```python
from build123d import *

# Parameters (mm, degrees)
SKETCH_W      = 60
SKETCH_H      = 3
PAD_DEPTH     = 35
SKETCH001_R   = 1.5
SKETCH001_R_2 = 2
SKETCH001_R_3 = 2.25
SKETCH001_R_4 = 1
SKETCH001_W   = 4
SKETCH001_H   = 7
POCKET_DEPTH  = 3


with BuildPart() as part:
    # Sketch → Pad (new body)
    with BuildSketch(Plane.XY):
        with Locations((30, 1.5)):
            Rectangle(SKETCH_W, SKETCH_H)
    extrude(amount=PAD_DEPTH)

    # Sketch001 → Pocket (cut)
    with BuildSketch(Plane.XZ):
        with Locations((22, 10)):
            Circle(SKETCH001_R)
        with Locations((28, 10)):
            Circle(SKETCH001_R_2)
        with Locations((22, 16)):
            Circle(SKETCH001_R_2)
        with Locations((16, 10)):
            Circle(SKETCH001_R_2)
        with Locations((22, 4)):
            Circle(SKETCH001_R_2)
        with Locations((5, 30)):
            Circle(SKETCH001_R_3)
        with Locations((55, 30)):
            Circle(SKETCH001_R_3)
        with Locations((14, 30)):
            Circle(SKETCH001_R_4)
        with Locations((18, 30)):
            Circle(SKETCH001_R_4)
        with Locations((26, 30)):
            Circle(SKETCH001_R_4)
        with Locations((30, 30)):
            Circle(SKETCH001_R_4)
        with Locations((34, 30)):
            Circle(SKETCH001_R_4)
        with Locations((42, 30)):
            Circle(SKETCH001_R_4)
        with Locations((46, 30)):
            Circle(SKETCH001_R_4)
        with Locations((45.6, 15)):
            Circle(SKETCH001_R)
        with Locations((45.6, 4.8)):
            Circle(SKETCH001_R)
        with Locations((22, 30)):
            Rectangle(SKETCH001_W, SKETCH001_H)
        with Locations((38, 30)):
            Rectangle(SKETCH001_W, SKETCH001_H)
    extrude(amount=-POCKET_DEPTH, mode=Mode.SUBTRACT)


solid = part.part
```
The listing builds one solid part. Answer for the finished solid, in the listing's coordinates (mm). A direction names the side the tool comes from. Coordinates: 2 decimals unless noted, no trailing zeros. Loops run counter-clockwise (first coordinate to the right, second up) from the corner with the lowest first, then second, coordinate; pieces in that order, holes last. Notation, with made-up numbers: (-17.75, 22) -> (14.25, 22) arc R11 ccw to (14.25, 32) -> close; hole circle Ø7 at (58, 21). An arc over 180 degrees is marked (long way). Use one line per item in the form item = value. Start each with the question number.
Item 1: The part is cut by section A-A on z = 10. Determine the outline of the cut face in (x, y), then the cut area to 3 significant figures.
Item 2: Consider L1, parallel to Z at x = 39.5, y = 1.25; L2, parallel to X at y = 2.4, z = 9; L3, parallel to Z at x = 46, y = 0.2. Determine where each line is inside the solid, lowest interval first. Write a range as [from, to].
Item 3: The mould has two halves that part along Z. Classify faces 1 (the face through (7.08, 1.48, 29.14)), 2 (the face through (30, 2, 0)), 3 (the face through (0, 1, 17)): released by +Z, released by -Z, zero draft, split by the parting line, or undercut.
Item 4: A tool of negligible diameter and unlimited length cuts with its end or side. For faces 4 (the face through (24, 1, 30)), 5 (the face through (60, 1, 17)), from which of +Z, -Z, +X, -X, +Y, -Y can it reach the whole face along a straight path? Write none if from no direction.
Item 5: The part is cut by section B-B on x = 38.5. Determine the outline of the cut face in (y, z), then the cut area to 3 significant figures.
Item 6: The part is cut by section D-D on x = 16. Determine the outline of the cut face in (y, z).
Item 7: The part is cut by section C-C on y = 0.85. Count the separate pieces of the cut face and the enclosed holes in it, then the cut area to 3 significant figures.
Answer key:
q1.outline = (0, 0) -> (14, 0) -> (14, 3) -> (0, 3) -> close; (18, 0) -> (20.5, 0) -> (20.5, 3) -> (18, 3) -> close; (23.5, 0) -> (26, 0) -> (26, 3) -> (23.5, 3) -> close; (30, 0) -> (60, 0) -> (60, 3) -> (30, 3) -> close
q1.area = 147 mm2
q2.L1 = [0, 26.5], [33.5, 35]
q2.L2 = [0, 14.27], [17.73, 20.88], [23.12, 26.27], [29.73, 60]
q2.L3 = [0, 3.35], [6.25, 13.55], [16.45, 29], [31, 35]
q3.face_1 = undercut
q3.face_2 = released by -Z
q3.face_3 = zero draft
q4.face_4 = +Y, -Y
q4.face_5 = +Z, -Z, +X, +Y, -Y
q5.outline = (0, 0) -> (3, 0) -> (3, 26.5) -> (0, 26.5) -> close; (0, 33.5) -> (3, 33.5) -> (3, 35) -> (0, 35) -> close
q5.area = 84.0 mm2
q6.outline = (0, 0) -> (3, 0) -> (3, 8) -> (0, 8) -> close; (0, 12) -> (3, 12) -> (3, 35) -> (0, 35) -> close
q7.separate_pieces = 1
q7.enclosed_holes = 18
q7.area = 1,920 mm2
